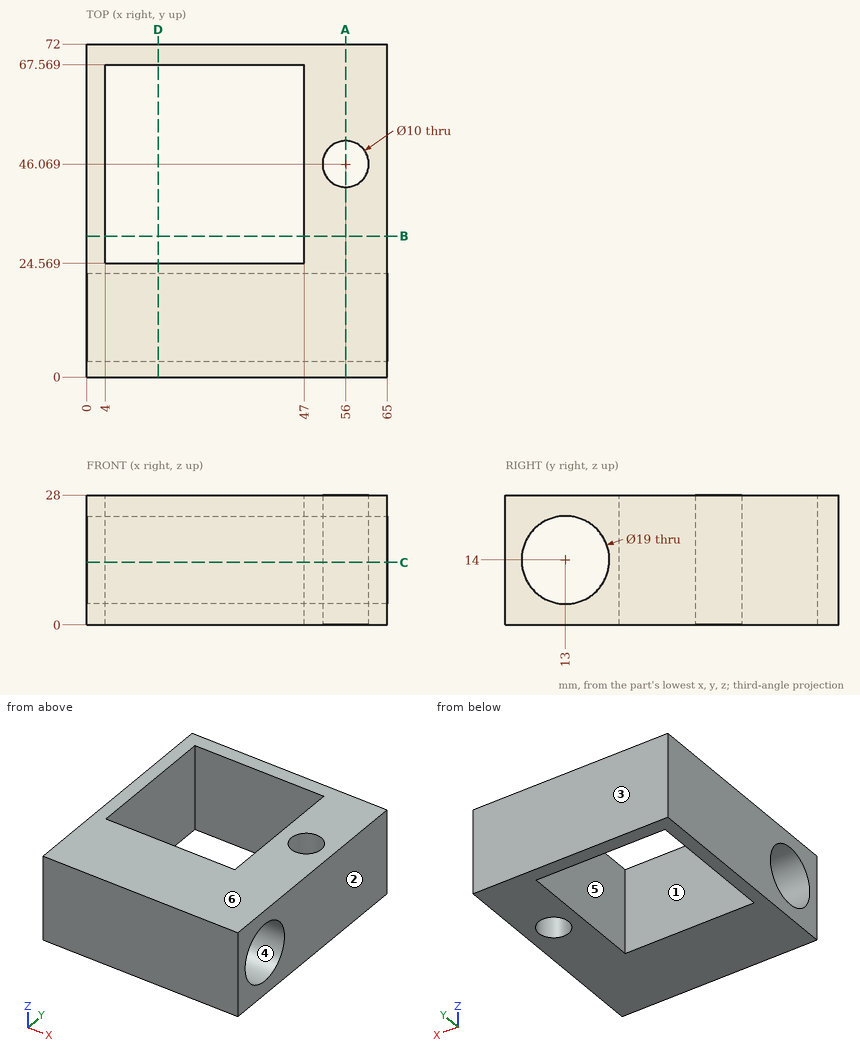
Answer from the drawing. Dimensions are ordinates in mm from the lowest x, y and z of the part. A direction names the side the tool comes from. Round coordinates to 2 decimals unless told otherwise and drop trailing zeros. Order: outer loops, then holes, each group sorted by start corner. A loop starts at its lowest first (then second) coordinate and runs counter-clockwise, first axis right, second up.
1) The part is cut by section C-C on z = 13.5. Write down the section's boundary in (x, y), plus the area to 3 significant figures.
2) Straight lines are drawn through the part: L1, parallel to Y at x = 28.5, z = 14; L2, parallel to X at y = 46.5, z = 14.25; L3, parallel to Y at x = 56, z = 13.75. For each, find the intervals that lie inside material, in ascending order.
3) A flat-ended cylindrical pin translates along its axis: pin 1 (5 mm diameter, centred on y = 27.5, z = 11, fed in from -X). Find the tip coordinate at first contact, or state that the pin passes through.
4) The mould has two halves that part along Y. Classify the marked faces 3, 4, 5 and 6: released by +Y, released by -Y, zero draft, split by the parting line, or undercut.
5) For the marked faces 1 and 2, determine the directions among +Z, -Z, +X, -X, +Y, -Y from which every point of the face is accessible in a straight line to the end or side of a thin tool.
6) The part is cut by section A-A on x = 56. Write down the section's boundary in (y, z).
7) The part is cut by section B-B on y = 30.5. Write down the section's boundary in (x, z).
8) The part is cut by section D-D on x = 15.5. Write down the section's boundary in (y, z).
Resolved:
1. outline: (0, 0) - (65, 0) - (65, 3.51) - (0, 3.51) - close; (0, 22.49) - (65, 22.49) - (65, 72) - (0, 72) - close; hole (4, 24.57) - (47, 24.57) - (47, 67.57) - (4, 67.57) - close; hole circle Ø10 at (56, 46.07)
1. area: 1,520 mm2
2. L1: y = 0 to 3.5, 22.5 to 24.57, 67.57 to 72
2. L2: x = 0 to 4, 47 to 51.02, 60.98 to 65
2. L3: y = 0 to 3.5, 22.5 to 41.07, 51.07 to 72
3. pin 1: stops at x = 0
4. face 3: released by +Y
4. face 4: undercut
4. face 5: undercut
4. face 6: zero draft
5. face 1: +Z, -Z
5. face 2: +Z, -Z, +X, +Y, -Y
6. outline: (0, 0) - (41.07, 0) - (41.07, 28) - (0, 28) - close; (51.07, 0) - (72, 0) - (72, 28) - (51.07, 28) - close; hole circle Ø19 at (13, 14)
7. outline: (0, 0) - (4, 0) - (4, 28) - (0, 28) - close; (47, 0) - (65, 0) - (65, 28) - (47, 28) - close
8. outline: (0, 0) - (24.57, 0) - (24.57, 28) - (0, 28) - close; (67.57, 0) - (72, 0) - (72, 28) - (67.57, 28) - close; hole circle Ø19 at (13, 14)
